The model under review builds one solid part; all positions refer to its coordinate system, in mm. Give positions to 0.01 mm unless a question says otherwise; leave off trailing zeros. Order: outer loops, then holes, each group sorted by start corner. A loop starts at its lowest first (then second) coordinate and runs counter-clockwise, first axis right, second up. Notation, with made-up numbers: (20, 13) - (40, 13) arc R33 cw to (40, 47) - close; hole circle Ø7 at (3.25, -34). An arc over 180 degrees is marked (long way). Answer as CSV lines item,"result". Start each with the question number.
from build123d import *

# Parameters (mm, degrees)
F0_W     = 50.8
F0_H     = 12.7
F1_DEPTH = 76.2
F2_SIZE  = 12.69999


# Not quite as in the source:
# - a fillet or chamfer is up to 0.001 mm smaller than in the source, because OpenCascade refuses the exact size


with BuildPart() as f1:
    # F0 (on Right) → F1 (new body, symmetric)
    with BuildSketch(Plane.YZ):
        Rectangle(F0_W, F0_H)
    extrude(amount=F1_DEPTH, both=True)

    # F2 (size 12.7 in the source; OpenCascade refuses exactly that, so slightly less here)
    f2_edges = [f1.edges().sort_by_distance(p)[0] for p in [
        (0, 25.4, 6.35),
        (-76.2, 0, 6.35),
        (0, -25.4, 6.35),
        (76.2, 0, 6.35),
    ]]
    chamfer(f2_edges, length=F2_SIZE)


solid = f1.part
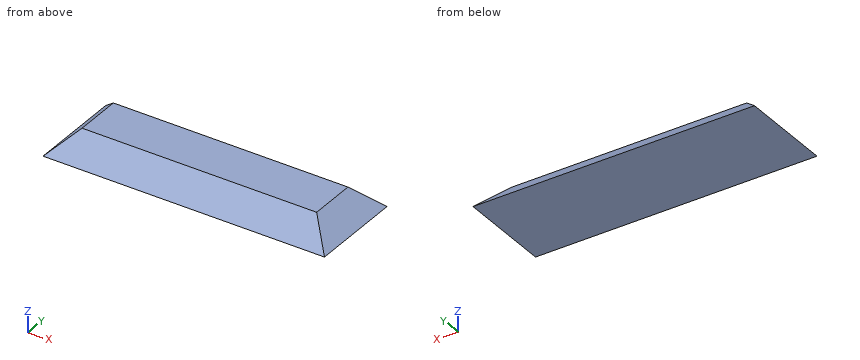
Item 1: Take a section at C-C on z = 1.75. Write out the cut boundary in (x, y).
Item 2: For line 1 along X through (y, z) = (1.5, 5); line 2 along Z through (x, y) = (51, -17); line 3 along Z through (x, y) = (31, 16), list the stretches that pass through material, from the lowest coordinate up.
Item 3: Clearance check with flat-ended pins moving along their axes: pin 1 (1 mm diameter, centred on y = -11.5, z = 1.5, fed in from +X); pin 2 (6 mm diameter, centred on y = 16.5, z = -3, fed in from +X); pin 3 (4 mm diameter, centred on x = -8, z = 3, fed in from +Y). State where each tip first meets the part, or that it passes through.
Item 4: Take a section at D-D on z = -5. Write out the cut boundary in (x, y).
Data:
1,outline,"(-68.1, -17.3) - (68.1, -17.3) - (68.1, 17.3) - (-68.1, 17.3) - close"
2,line 1,"x = -64.85 to 64.85"
2,line 2,"z = -6.35 to 2.05"
2,line 3,"z = -6.35 to 3.05"
3,pin 1,"stops at x = 68.85"
3,pin 2,"stops at x = 75.85"
3,pin 3,"stops at y = 18.05"
4,outline,"(-74.85, -24.05) - (74.85, -24.05) - (74.85, 24.05) - (-74.85, 24.05) - close"
